Could you check a few things on this model? Use its own coordinates, in mm. A direction names the side the tool comes from. Round coordinates to 2 decimals unless told otherwise and drop trailing zeros. Order: outer loops, then holes, each group sorted by start corner. A loop starts at its lowest first (then second) coordinate and runs counter-clockwise, first axis right, second up. Notation, with made-up numbers: (34.25, 13.5) - (79.25, 13.5) arc R5 cw to (79.25, 22.5) - close; hole circle Ø4 at (11.25, 38). An arc over 180 degrees is marked (long way). Return JSON: item names as keys, results as strings. Group by question number.
from build123d import *

# Parameters (mm, degrees)
SKETCH1_R               = 4.5
SKETCH1_R_2             = 2
BOSS_EXTRUDE1_DEPTH     = 10
CHAMFER1_SIZE           = 2
CHAMFER1_SIZE2          = 3.464101615
SKETCH2_R               = 2.25
CUT_EXTRUDE2_DEPTH      = 3.6
CUT_EXTRUDE3_DEPTH      = 12.853269591
CUT_EXTRUDE3_DEPTH_BACK = 12.853269591
SKETCH3_R               = 8
CHAMFER2_SIZE           = 0.2


with BuildPart() as part:
    # Sketch1 → Boss-Extrude1 (new body)
    with BuildSketch(Plane(origin=(0, 0, 0), x_dir=(1, 0, 0), z_dir=(0, 1, 0))):
        with Locations(Location((0, 0, 0), (0, 0, 270))):
            Circle(SKETCH1_R)
        with Locations(Location((0, 0, 0), (0, 0, 270))):
            Circle(SKETCH1_R_2, mode=Mode.SUBTRACT)
    extrude(amount=BOSS_EXTRUDE1_DEPTH)

    # Chamfer1
    chamfer1_edges = [part.edges().sort_by_distance(p)[0] for p in [
        (0, 10, -2),
    ]]
    chamfer1_side = [part.faces().sort_by_distance(p)[0] for p in [
        (0, 10, -4.372720779),
    ]]
    chamfer(chamfer1_edges, length=CHAMFER1_SIZE, length2=CHAMFER1_SIZE2, reference=chamfer1_side[0])

    # Sketch2 → Cut-Extrude2 (cut)
    with BuildSketch(Plane.XZ):
        with Locations(Location((0, 0, 0), (0, 0, 270))):
            Circle(SKETCH2_R)
    extrude(amount=-CUT_EXTRUDE2_DEPTH, mode=Mode.SUBTRACT)

    # Sketch3 → Cut-Extrude3 (cut, two sides: drawn at the far end of the back side and taken through both)
    with BuildSketch(Plane.XY.offset(-CUT_EXTRUDE3_DEPTH_BACK)):
        with Locations((7, 12)):
            Circle(SKETCH3_R)
    extrude(amount=CUT_EXTRUDE3_DEPTH + CUT_EXTRUDE3_DEPTH_BACK, mode=Mode.SUBTRACT)

    # Chamfer2
    chamfer2_edges = [part.edges().sort_by_distance(p)[0] for p in [
        (0, 3.6, -2),
        (0, 0, 2.25),
    ]]
    chamfer(chamfer2_edges, length=CHAMFER2_SIZE)


solid = part.part
1) We'd pull the mould along Z, two halves only. Please class faces 1 (the cylindrical face through (-2, 5, 0)), 2 (the cylindrical face through (-4.39, 3.82, -0.98)), 3 (the flat face through (-2, 0, 2)): +Z half, -Z half, draft (parallel to the pull), parting line (faces both ways), or undercut.
2) I want a section at A-A, the plane z = 0. List the corners of the cut face in (x, y) for me (3 decimals).
3) I want a section at D-D, the plane x = 3. List the corners of the cut face in (y, z) for me.
4) I want a section at B-B, the plane x = 0. List the corners of the cut face in (y, z) for me, plus the area to 3 significant figures.
5) If I drill on line 1 along X through (y, z) = (1.45, 0); line 2 along Z through (x, y) = (0, 5.6); line 3 along X through (y, z) = (5.55, 0), over which ranges is the centre line in solid material (lowest first)? Write a range as from..to.
6) For faces 4 (the cylindrical face through (2.465, 5.409, -0.07)), 5 (the cylindrical face through (0.676, 1.876, -2.146)), which set-ups out of +Z, -Z, +X, -X, +Y, -Y let a thin tool reach every point of the face, with its end or its side?
7) I want a section at C-C, the plane y = 1.75. List the corners of the cut face in (x, z) for me.
8) Will these pins go through, and if not, where does the flat tip stop? pin 1 (5 mm diameter, centred on x = 0, z = 0, fed in from +Y); pin 2 (1 mm diameter, centred on x = 0.5, z = 1.5, fed in from -Y).
Outcome:
{
 "1": {"face 1": "undercut", "face 2": "parting line", "face 3": "draft"},
 "2": {"outline": "(-4.5, 0) - (-2.45, 0) - (-2.25, 0.2) - (-2.25, 3.6) - (-2.2, 3.6) - (-2, 3.8) - (-2, 6.536) - (-4, 10) - (-4.5, 10) - close; (2, 3.8) - (2.2, 3.6) - (2.25, 3.6) - (2.25, 0.2) - (2.45, 0) - (4.5, 0) - (4.5, 4.401) arc R8 cw to (2, 5.755) - close"},
 "3": {"outline": "(0, -3.35) - (5.07, -3.35) - (5.07, 3.35) - (0, 3.35) - close"},
 "4": {"outline": "(0, -4.5) - (8.13, -4.5) - (8.13, -2.92) - (6.54, -2) - (3.8, -2) - (3.6, -2.2) - (3.6, -2.25) - (0.2, -2.25) - (0, -2.45) - close; (0, 2.45) - (0.2, 2.25) - (3.6, 2.25) - (3.6, 2.2) - (3.8, 2) - (6.54, 2) - (8.13, 2.92) - (8.13, 4.5) - (0, 4.5) - close", "area": "37.3 mm^2"},
 "5": {"line 1": "-4.5..-2.25, 2.25..4.5", "line 2": "-4.5..-2, 2..4.5", "line 3": "-4.5..-2, 2..2.27"},
 "6": {"face 4": "+Z, -Z, +X, +Y", "face 5": "-Y"},
 "7": {"outline": "circle Ø9 at (0, 0); hole circle Ø4.5 at (0, 0)"},
 "8": {"pin 1": "y = 7.4", "pin 2": "y = 3.72"}
}
